The model under review builds one solid part; all positions refer to its coordinate system, in mm. Face numbers are marked on the shaded views. A direction names the side the tool comes from. Coordinates: 2 decimals unless noted, no trailing zeros. Order: outer loops, then holes, each group sorted by start corner. A loop starts at its lowest first (then second) coordinate and runs counter-clockwise, first axis right, second up.
```python
from build123d import *

# Parameters (mm, degrees)
SKETCH_W        = 12.5
SKETCH_H        = 6
PAD001_DEPTH    = 6
SKETCH006_W     = 3.8
SKETCH006_H     = 3.8
PAD002_DEPTH    = 8
CHAMFER_1_ANGLE = 60
CHAMFER_1_SIZE  = 0.5
CHAMFER_2_ANGLE = 60
CHAMFER_2_SIZE  = 0.5


with BuildPart() as part:
    # Sketch → Pad001 (new body)
    with BuildSketch(Plane.XY):
        Rectangle(SKETCH_W, SKETCH_H)
    extrude(amount=PAD001_DEPTH)

    # Sketch006 → Pad002 (join)
    with BuildSketch(Plane.XZ):
        with Locations((1.35, 3)):
            Rectangle(SKETCH006_W, SKETCH006_H)
    extrude(amount=-PAD002_DEPTH)

    # Chamfer 1
    chamfer_1_edges = [part.edges().sort_by_distance(p)[0] for p in [
        (3.25, 8, 3),
    ]]
    chamfer_1_side = part.faces().sort_by_distance((3.25, 5.5, 3))[0]
    chamfer(chamfer_1_edges, length=CHAMFER_1_SIZE, angle=CHAMFER_1_ANGLE, reference=chamfer_1_side)

    # Chamfer 2
    chamfer_2_edges = [part.edges().sort_by_distance(p)[0] for p in [
        (-0.55, 8, 3),
    ]]
    chamfer_2_side = part.faces().sort_by_distance((-0.55, 5.5, 3))[0]
    chamfer(chamfer_2_edges, length=CHAMFER_2_SIZE, angle=CHAMFER_2_ANGLE, reference=chamfer_2_side)


solid = part.part
```
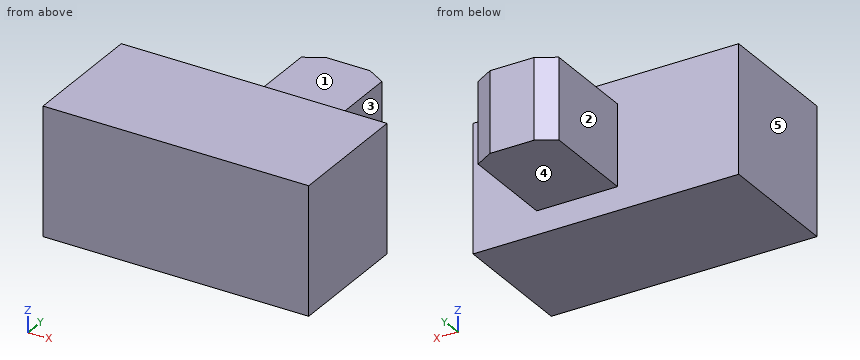
(1) Wall thickness on probe 1 along Y at (x, z) = (3.5, 3.9); probe 2 along Z at (x, y) = (1.25, 7); probe 3 along X at (y, z) = (4.75, 1.45): over which ranges is each line inside the solid? List them lowest first.
A:
probe 1: y = -3 to 3
probe 2: z = 1.1 to 4.9
probe 3: x = -0.55 to 3.25
(2) Machinability: for the marked faces 1, 2, 3, 4 and 5, which of the approach directions +Z, -Z, +X, -X, +Y, -Y give a long, thin tool a straight path to every point of the face, cutting with its end or side? Answer none if there is none.
A:
face 1: +Z, +X, -X, +Y
face 2: +Z, -Z, -X, +Y
face 3: +Z, -Z, +X, +Y
face 4: -Z, +X, -X, +Y
face 5: +Z, -Z, -X, +Y, -Y
(3) We need section B-B, the plane x = 5. Write out the cut boundary in (y, z), and give its area (3 significant figures).
A:
outline: (-3, 0) - (3, 0) - (3, 6) - (-3, 6) - close
area: 36.0 mm2
(4) We need section C-C, the plane y = 4.5. Write out the cut boundary in (x, z).
A:
outline: (-0.55, 1.1) - (3.25, 1.1) - (3.25, 4.9) - (-0.55, 4.9) - close
(5) We need section A-A, the plane z = 2.55. Write out the cut boundary in (x, y).
A:
outline: (-6.25, -3) - (6.25, -3) - (6.25, 3) - (3.25, 3) - (3.25, 7.5) - (2.38, 8) - (0.32, 8) - (-0.55, 7.5) - (-0.55, 3) - (-6.25, 3) - close
(6) For pin 1 Ø1.1 at (y, z) = (5, 3.5) entering from +X; pin 2 Ø3 at (x, z) = (4, 3) entering from +Y; pin 3 Ø1.1 at (x, y) = (1, 6) entering from -Z, all flat-tipped, find the tip position at first contact; note any pin that passes through.
A:
pin 1: stops at x = 3.25
pin 2: stops at y = 7.93
pin 3: stops at z = 1.1
(7) We need section D-D, the plane x = -0.25. Write out the cut boundary in (y, z).
A:
outline: (-3, 0) - (3, 0) - (3, 1.1) - (7.67, 1.1) - (7.67, 4.9) - (3, 4.9) - (3, 6) - (-3, 6) - close
